from build123d import *

# Parameters (mm, degrees)
BOSS_EXTRUDE2_DEPTH = 125
SKETCH2_W           = 51.623637996
SKETCH2_H           = 2
BOSS_EXTRUDE3_DEPTH = 12
SKETCH3_W           = 5
SKETCH3_H           = 10
BOSS_EXTRUDE4_DEPTH = 11
CUT_EXTRUDE1_REACH  = 16.942
SKETCH4_R           = 1.3


with BuildPart() as part:
    # Model → Boss-Extrude2 (new body)
    with BuildSketch(Plane.XY):
        with BuildLine():
            ThreePointArc((25.811818998, 6), (24.648760727, 9.730806474), (22.9496732, 13.25))
            Line((22.9496732, 13.25), (21.650635095, 12.5))
            ThreePointArc((21.650635095, 12.5), (22.886510643, 10.060200326), (23.848480035, 7.5))
            ThreePointArc((23.848480035, 7.5), (24.070588339, 6.753278984), (24.269322199, 6))
            Line((24.269322199, 6), (25.811818998, 6))
        make_face()
        with BuildLine():
            ThreePointArc((24.269322199, 6), (24.070588339, 6.753278984), (23.848480035, 7.5))
            Line((23.848480035, 7.5), (23.323807579, 7.5))
            Line((23.323807579, 7.5), (21.213203436, 7.5))
            Line((21.213203436, 7.5), (20.68211788, 7.5))
            ThreePointArc((20.68211788, 7.5), (20.937501331, 6.754334757), (21.166010489, 6))
            Line((21.166010489, 6), (24.269322199, 6))
        make_face()
        with BuildLine():
            Line((19.602295784, 6), (21.166010489, 6))
            ThreePointArc((21.166010489, 6), (20.937501331, 6.754334757), (20.68211788, 7.5))
            ThreePointArc((20.68211788, 7.5), (19.944263194, 9.285815292), (19.052558883, 11))
            Line((19.052558883, 11), (17.753520778, 10.25))
            ThreePointArc((17.753520778, 10.25), (18.798401069, 8.177415072), (19.602295784, 6))
        make_face()
        with BuildLine():
            Line((10.392304845, 6), (19.602295784, 6))
            ThreePointArc((19.602295784, 6), (18.798401069, 8.177415072), (17.753520778, 10.25))
            Line((17.753520778, 10.25), (10.392304845, 6))
        make_face()
        Polygon((17.753520778, 10.25), (-17.753520778, 10.25), (-10.392304845, 6), (10.392304845, 6), align=None)
        with BuildLine():
            Line((-17.753520778, 10.25), (-19.052558883, 11))
            ThreePointArc((-19.052558883, 11), (-19.944263194, 9.285815292), (-20.68211788, 7.5))
            ThreePointArc((-20.68211788, 7.5), (-20.937501331, 6.754334757), (-21.166010489, 6))
            Line((-21.166010489, 6), (-19.602295784, 6))
            ThreePointArc((-19.602295784, 6), (-18.798401069, 8.177415072), (-17.753520778, 10.25))
        make_face()
        with BuildLine():
            Line((-21.213203436, 7.5), (-23.323807579, 7.5))
            ThreePointArc((-23.323807579, 7.5), (-23.550822597, 6.753425426), (-23.75394704, 6))
            Line((-23.75394704, 6), (-21.685248442, 6))
            ThreePointArc((-21.685248442, 6), (-21.462334295, 6.754125156), (-21.213203436, 7.5))
        make_face()
        with BuildLine():
            Line((-23.323807579, 7.5), (-23.848480035, 7.5))
            ThreePointArc((-23.848480035, 7.5), (-24.070588339, 6.753278984), (-24.269322199, 6))
            Line((-24.269322199, 6), (-23.75394704, 6))
            ThreePointArc((-23.75394704, 6), (-23.550822597, 6.753425426), (-23.323807579, 7.5))
        make_face()
        with BuildLine():
            Line((-20.68211788, 7.5), (-21.213203436, 7.5))
            ThreePointArc((-21.213203436, 7.5), (-21.462334295, 6.754125156), (-21.685248442, 6))
            Line((-21.685248442, 6), (-21.166010489, 6))
            ThreePointArc((-21.166010489, 6), (-20.937501331, 6.754334757), (-20.68211788, 7.5))
        make_face()
        with BuildLine():
            Line((-21.650635095, 12.5), (-22.9496732, 13.25))
            ThreePointArc((-22.9496732, 13.25), (-24.648760727, 9.730806474), (-25.811818998, 6))
            Line((-25.811818998, 6), (-24.269322199, 6))
            ThreePointArc((-24.269322199, 6), (-24.070588339, 6.753278984), (-23.848480035, 7.5))
            ThreePointArc((-23.848480035, 7.5), (-22.886510643, 10.060200326), (-21.650635095, 12.5))
        make_face()
        with BuildLine():
            Line((-10.392304845, 6), (-17.753520778, 10.25))
            ThreePointArc((-17.753520778, 10.25), (-18.798401069, 8.177415072), (-19.602295784, 6))
            Line((-19.602295784, 6), (-10.392304845, 6))
        make_face()
        with BuildLine():
            Line((-24.269322199, -6), (-25.811818998, -6))
            ThreePointArc((-25.811818998, -6), (-24.648760727, -9.730806474), (-22.9496732, -13.25))
            Line((-22.9496732, -13.25), (-21.650635095, -12.5))
            ThreePointArc((-21.650635095, -12.5), (-22.886510643, -10.060200326), (-23.848480035, -7.5))
            ThreePointArc((-23.848480035, -7.5), (-24.070588339, -6.753278984), (-24.269322199, -6))
        make_face()
        with BuildLine():
            Line((-23.75394704, -6), (-24.269322199, -6))
            ThreePointArc((-24.269322199, -6), (-24.070588339, -6.753278984), (-23.848480035, -7.5))
            Line((-23.848480035, -7.5), (-23.323807579, -7.5))
            ThreePointArc((-23.323807579, -7.5), (-23.550822597, -6.753425426), (-23.75394704, -6))
        make_face()
        with BuildLine():
            Line((-21.685248442, -6), (-23.75394704, -6))
            ThreePointArc((-23.75394704, -6), (-23.550822597, -6.753425426), (-23.323807579, -7.5))
            Line((-23.323807579, -7.5), (-21.213203436, -7.5))
            ThreePointArc((-21.213203436, -7.5), (-21.462334295, -6.754125156), (-21.685248442, -6))
        make_face()
        with BuildLine():
            Line((-21.166010489, -6), (-21.685248442, -6))
            ThreePointArc((-21.685248442, -6), (-21.462334295, -6.754125156), (-21.213203436, -7.5))
            Line((-21.213203436, -7.5), (-20.68211788, -7.5))
            ThreePointArc((-20.68211788, -7.5), (-20.937501331, -6.754334757), (-21.166010489, -6))
        make_face()
        with BuildLine():
            Line((-19.602295784, -6), (-21.166010489, -6))
            ThreePointArc((-21.166010489, -6), (-20.937501331, -6.754334757), (-20.68211788, -7.5))
            ThreePointArc((-20.68211788, -7.5), (-19.944263194, -9.285815292), (-19.052558883, -11))
            Line((-19.052558883, -11), (-17.753520778, -10.25))
            ThreePointArc((-17.753520778, -10.25), (-18.798401069, -8.177415072), (-19.602295784, -6))
        make_face()
        with BuildLine():
            Line((-17.753520778, -10.25), (-10.392304845, -6))
            Line((-10.392304845, -6), (-19.602295784, -6))
            ThreePointArc((-19.602295784, -6), (-18.798401069, -8.177415072), (-17.753520778, -10.25))
        make_face()
        Polygon((17.753520778, -10.25), (10.392304845, -6), (-10.392304845, -6), (-17.753520778, -10.25), align=None)
        with BuildLine():
            ThreePointArc((17.753520778, -10.25), (18.798401069, -8.177415072), (19.602295784, -6))
            Line((19.602295784, -6), (10.392304845, -6))
            Line((10.392304845, -6), (17.753520778, -10.25))
        make_face()
        with BuildLine():
            ThreePointArc((20.68211788, -7.5), (20.937501331, -6.754334757), (21.166010489, -6))
            Line((21.166010489, -6), (19.602295784, -6))
            ThreePointArc((19.602295784, -6), (18.798401069, -8.177415072), (17.753520778, -10.25))
            Line((17.753520778, -10.25), (19.052558883, -11))
            ThreePointArc((19.052558883, -11), (19.944263194, -9.285815292), (20.68211788, -7.5))
        make_face()
        with BuildLine():
            ThreePointArc((23.848480035, -7.5), (24.070588339, -6.753278984), (24.269322199, -6))
            Line((24.269322199, -6), (21.166010489, -6))
            ThreePointArc((21.166010489, -6), (20.937501331, -6.754334757), (20.68211788, -7.5))
            Line((20.68211788, -7.5), (21.213203436, -7.5))
            Line((21.213203436, -7.5), (23.323807579, -7.5))
            Line((23.323807579, -7.5), (23.848480035, -7.5))
        make_face()
        with BuildLine():
            ThreePointArc((22.9496732, -13.25), (24.648760727, -9.730806474), (25.811818998, -6))
            Line((25.811818998, -6), (24.269322199, -6))
            ThreePointArc((24.269322199, -6), (24.070588339, -6.753278984), (23.848480035, -7.5))
            ThreePointArc((23.848480035, -7.5), (22.886510643, -10.060200326), (21.650635095, -12.5))
            Line((21.650635095, -12.5), (22.9496732, -13.25))
        make_face()
    extrude(amount=BOSS_EXTRUDE2_DEPTH)

    # Sketch2 → Boss-Extrude3 (add)
    with BuildSketch(Plane.XZ.offset(-6)):
        with Locations((0, 1)):
            Rectangle(SKETCH2_W, SKETCH2_H)
    extrude(amount=BOSS_EXTRUDE3_DEPTH)

    # Sketch3 → Boss-Extrude4 (add)
    with BuildSketch(Plane(origin=(0, 0, 0), x_dir=(-1, 0, 0), z_dir=(0, 0, -1))):
        with Locations((-13.5, -3.307781384)):
            Rectangle(SKETCH3_W, SKETCH3_H)
        with Locations((13.5, -3.307781384)):
            Rectangle(SKETCH3_W, SKETCH3_H)
    extrude(amount=BOSS_EXTRUDE4_DEPTH)

    # Sketch4 → Cut-Extrude1 (cut, up to next)
    with BuildSketch(Plane(origin=(0, 1.692218616, 0), x_dir=(1, 0, 0), z_dir=(0, 1, 0)), mode=Mode.PRIVATE) as cut_extrude1_sk1:
        with Locations((14, 5.5)):
            Circle(SKETCH4_R)
    cut_extrude1_tool1 = extrude(cut_extrude1_sk1.sketch, amount=-CUT_EXTRUDE1_REACH, mode=Mode.PRIVATE) & part.part
    add(cut_extrude1_tool1.solids().sort_by_distance((14, 1.692219, -5.5))[0], mode=Mode.SUBTRACT)
    # Sketch4 → Cut-Extrude1 (cut, up to next)
    with BuildSketch(Plane(origin=(0, 1.692218616, 0), x_dir=(1, 0, 0), z_dir=(0, 1, 0)), mode=Mode.PRIVATE) as cut_extrude1_sk2:
        with Locations((-14, 5.5)):
            Circle(SKETCH4_R)
    cut_extrude1_tool2 = extrude(cut_extrude1_sk2.sketch, amount=-CUT_EXTRUDE1_REACH, mode=Mode.PRIVATE) & part.part
    add(cut_extrude1_tool2.solids().sort_by_distance((-14, 1.692219, -5.5))[0], mode=Mode.SUBTRACT)


solid = part.part
Build history of the part. All positions in model axes, mm. A direction names the side the tool comes from. Round coordinates to 2 decimals unless told otherwise and drop trailing zeros. Loops run counter-clockwise (first coordinate to the right, second up) from the corner with the lowest first, then second, coordinate; pieces in that order, holes last. Notation, with made-up numbers: (85, -28) -> (120, -28) arc R20 ccw to (120, 7) -> close; hole circle Ø6 at (63, 82.5). An arc over 180 degrees is marked (long way). One line per item, written item: value. Start each with the question number.
Q1. Drop flat-ended pins along their axis: pin 1 Ø6 at (y, z) = (-6, 105) entering from +X; pin 2 Ø6 at (x, y) = (7, 0) entering from -Z; pin 3 Ø1.6 at (x, z) = (22, 66.5) entering from -Y; pin 4 Ø8 at (x, y) = (-19, -0.5) entering from -Z. Give the stop position or say it passes through.
Q2. Two-plate mould, pull along X, no slides. Class faces 4 (the face through (-24.63, 9.78, 61.62)), 5 (the face through (-22.9, 10.03, 61.62)), 6 (the face through (-13, -3, -11)): released by +X, released by -X, zero draft, split by the parting line, or undercut.
Q3. 3-axis set-ups, long thin cutter, end or side, ignore diameter. For faces 1 (the face through (11, -3, -5)), 2 (the face through (12, -8.308, -5)), 3 (the face through (19.933, -9.31, 61.625)): which of +Z, -Z, +X, -X, +Y, -Y reach the whole face in a straight line?
Q4. Cut at B-B on z = -5.5. List the corners of the cut face in (x, y), plus the area to 3 significant figures.
Q5. Cut at D-D on z = 41. List the corners of the cut face in (x, y), plus the area to 3 significant figures.
Q6. Probe line 1 along X through (y, z) = (-4.75, -5.5); line 2 along Y through (x, z) = (-21.5, 105.5); line 3 along Y through (x, z) = (-10.5, 4). List the from-to ranges inside material, lowest first.
Q7. Cut at C-C on x = 14. List the corners of the cut face in (y, z), plus the area to 3 significant figures.
Q8. Cut at A-A on y = 0. List the corners of the cut face in (x, z).
Computed:
1. pin 1: x = 25.81
1. pin 2: z = 0
1. pin 3: y = -13.16
1. pin 4: z = -11
2. face 4: released by -X
2. face 5: undercut
2. face 6: zero draft
3. face 1: -Z, +Y, -Y
3. face 2: -Z, +X, -X, -Y
3. face 3: +Z, -Z, -Y
4. outline: (-16, -8.31) -> (-15.3, -8.31) -> (-15.3, 1.69) -> (-16, 1.69) -> close; (-12.7, -8.31) -> (-11, -8.31) -> (-11, 1.69) -> (-12.7, 1.69) -> close; (11, -8.31) -> (12.7, -8.31) -> (12.7, 1.69) -> (11, 1.69) -> close; (15.3, -8.31) -> (16, -8.31) -> (16, 1.69) -> (15.3, 1.69) -> close
4. area: 48.0 mm²
5. outline: (-25.81, -6) arc R26.5 ccw to (-22.95, -13.25) -> (-21.65, -12.5) arc R25 cw to (-23.85, -7.5) -> (-20.68, -7.5) arc R22 ccw to (-19.05, -11) -> (-17.75, -10.25) -> (17.75, -10.25) -> (19.05, -11) arc R22 ccw to (20.68, -7.5) -> (23.85, -7.5) arc R25 cw to (21.65, -12.5) -> (22.95, -13.25) arc R26.5 ccw to (25.81, -6) -> close; (-25.81, 6) -> (25.81, 6) arc R26.5 ccw to (22.95, 13.25) -> (21.65, 12.5) arc R25 cw to (23.85, 7.5) -> (20.68, 7.5) arc R22 ccw to (19.05, 11) -> (17.75, 10.25) -> (-17.75, 10.25) -> (-19.05, 11) arc R22 ccw to (-20.68, 7.5) -> (-23.85, 7.5) arc R25 cw to (-21.65, 12.5) -> (-22.95, 13.25) arc R26.5 ccw to start
5. area: 413 mm²
6. line 1: -16 to -15.3, -12.7 to -11, 11 to 12.7, 15.3 to 16
6. line 2: -7.5 to -6, 6 to 7.5
6. line 3: -10.25 to -6, 6 to 10.25
7. outline: (-10.25, 0) -> (-8.31, 0) -> (-8.31, -4.2) -> (1.69, -4.2) -> (1.69, 0) -> (10.25, 0) -> (10.25, 125) -> (6, 125) -> (6, 2) -> (-6, 2) -> (-6, 125) -> (-10.25, 125) -> close; (-8.31, -11) -> (1.69, -11) -> (1.69, -6.8) -> (-8.31, -6.8) -> close
7. area: 1,170 mm²
8. outline: (-25.81, 0) -> (-16, 0) -> (-16, -11) -> (-11, -11) -> (-11, 0) -> (11, 0) -> (11, -11) -> (16, -11) -> (16, 0) -> (25.81, 0) -> (25.81, 2) -> (-25.81, 2) -> close; hole circle Ø2.6 at (-14, -5.5); hole circle Ø2.6 at (14, -5.5)
